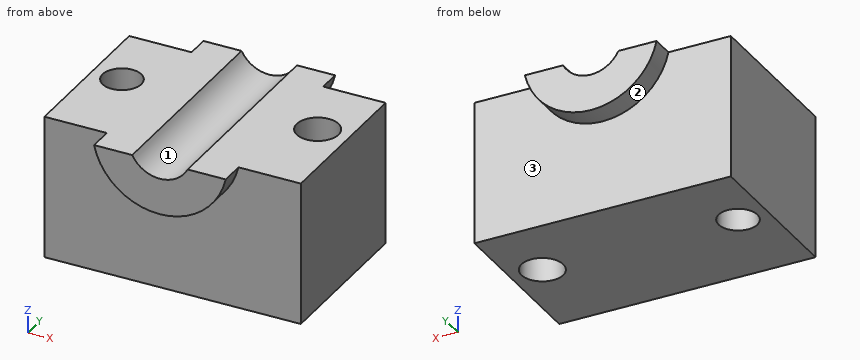
from build123d import *

# Parameters (mm, degrees)
F0_W          = 120.6022500992
F0_H          = 73.8097429276
F1_DEPTH      = 76.2
F2_R          = 31.6774975882
F3_DEPTH      = 86.868
F3_DEPTH_BACK = 11.43
F4_W          = 119.1478464752
F4_H          = 40.1731412858
F5_DEPTH      = 60.3021250496
F5_DEPTH_BACK = 60.3021250496
F6_R          = 14.6367961648
F7_DEPTH      = 86.869
F7_DEPTH_BACK = 25.4
F8_R          = 9.1115926715
F8_R_2        = 9.8364729175
F9_DEPTH      = 30.6065564433
F9_DEPTH_BACK = 36.9058714638


with BuildPart() as f1:
    # F0 (on Front) → F1 (new body)
    with BuildSketch(Plane.XZ):
        Rectangle(F0_W, F0_H)
    extrude(amount=-F1_DEPTH)

    # F2 (on Front) → F3 (join, two sides)
    with BuildSketch(Plane.XZ) as f3_sk:
        with Locations((0, 37.2918173671)):
            Circle(F2_R)
    extrude(amount=-F3_DEPTH)
    extrude(f3_sk.sketch, amount=F3_DEPTH_BACK)

    # F4 (on Right) → F5 (cut, two sides)
    with BuildSketch(Plane.YZ) as f5_sk:
        with Locations((41.5653018281, 50.6921270862)):
            Rectangle(F4_W, F4_H)
    extrude(amount=-F5_DEPTH, mode=Mode.SUBTRACT)
    extrude(f5_sk.sketch, amount=F5_DEPTH_BACK, mode=Mode.SUBTRACT)

    # F6 (on Front) → F7 (cut, two sides)
    with BuildSketch(Plane.XZ) as f7_sk:
        with Locations((0, 37.2918173671)):
            Circle(F6_R)
    extrude(amount=-F7_DEPTH, mode=Mode.SUBTRACT)
    extrude(f7_sk.sketch, amount=F7_DEPTH_BACK, mode=Mode.SUBTRACT)

    # F8 (on Top) → F9 (cut, two sides)
    with BuildSketch(Plane.XY) as f9_sk:
        with Locations((-46.2026000023, 42.7655205131)):
            Circle(F8_R)
        with Locations((45.4613789916, 43.5067377985)):
            Circle(F8_R_2)
    extrude(amount=F9_DEPTH, mode=Mode.SUBTRACT)
    extrude(f9_sk.sketch, amount=-F9_DEPTH_BACK, mode=Mode.SUBTRACT)


solid = f1.part
CAD build for the part. Positions are in the model's coordinates, mm. Face numbers are marked on the shaded views. Give positions to 0.01 mm unless a question says otherwise; leave off trailing zeros. Write each loop counter-clockwise with the first axis right and the second up, starting at its lowest first coordinate (ties: lowest second). Pieces come first, ordered by that corner, then holes. Notation, with made-up numbers: (82.5, -37) -> (107.5, -37) arc R24 cw to (107.5, -27) -> close; hole circle Ø1 at (42.25, -39.5). An arc over 180 degrees is marked (long way). Return JSON: item names as keys, results as strings.
Item 1: Band-saw the part on A-A (z = 26). List the corners of the cut face in (x, y), then the cut area to 3 significant figures.
Answer below:
{"outline": "(-60.3, 0) -> (-29.6, 0) -> (-29.6, -11.43) -> (-9.31, -11.43) -> (-9.31, 86.87) -> (-29.6, 86.87) -> (-29.6, 76.2) -> (-60.3, 76.2) -> close; (9.31, -11.43) -> (29.6, -11.43) -> (29.6, 0) -> (60.3, 0) -> (60.3, 76.2) -> (29.6, 76.2) -> (29.6, 86.87) -> (9.31, 86.87) -> close; hole circle Ø18.22 at (-46.2, 42.77); hole circle Ø19.67 at (45.46, 43.51)", "area": "8,100 mm2"}
Item 2: Band-saw the part on D-D (z = 15). List the corners of the cut face in (x, y), then the cut area to 3 significant figures.
Answer below:
{"outline": "(-60.3, 0) -> (-22.51, 0) -> (-22.51, -11.43) -> (22.51, -11.43) -> (22.51, 0) -> (60.3, 0) -> (60.3, 76.2) -> (22.51, 76.2) -> (22.51, 86.87) -> (-22.51, 86.87) -> (-22.51, 76.2) -> (-60.3, 76.2) -> close; hole circle Ø18.22 at (-46.2, 42.77); hole circle Ø19.67 at (45.46, 43.51)", "area": "9,620 mm2"}
Item 3: Band-saw the part on C-C (x = 0). List the corners of the cut face in (y, z), then the cut area to 3 significant figures.
Answer below:
{"outline": "(-11.43, 5.61) -> (0, 5.61) -> (0, -36.9) -> (76.2, -36.9) -> (76.2, 5.61) -> (86.87, 5.61) -> (86.87, 22.66) -> (-11.43, 22.66) -> close", "area": "4,920 mm2"}
Item 4: Drop flat-ended pins along their axis: pin 1 (11 mm diameter, centred on x = -46.2, y = 42.77, fed in from +Z); pin 2 (2 mm diameter, centred on x = 7, y = 22, fed in from +Z); pin 3 (6 mm diameter, centred on x = -3.5, z = -19, fed in from -Y); pin 4 (12 mm diameter, centred on x = 8, z = 6.5, fed in from +Y). Give the stop position or say it passes through.
Answer below:
{"pin 1": "passes through", "pin 2": "stops at z = 25.03", "pin 3": "stops at y = 0", "pin 4": "stops at y = 86.87"}
Item 5: Band-saw the part on B-B (y = 48.5). List the corners of the cut face in (x, z), then the cut area to 3 significant figures.
Answer below:
{"outline": "(-60.3, -36.9) -> (-53.28, -36.9) -> (-53.28, 30.61) -> (-60.3, 30.61) -> close; (-39.12, -36.9) -> (36.99, -36.9) -> (36.99, 30.61) -> (13.02, 30.61) arc R14.64 cw to (-13.02, 30.61) -> (-39.12, 30.61) -> close; (53.94, -36.9) -> (60.3, -36.9) -> (60.3, 30.61) -> (53.94, 30.61) -> close", "area": "5,890 mm2"}
Item 6: Two-plate mould, pull along X, no slides. Class the marked faces 1, 2 and 3: +X half, -X half, draft (parallel to the pull), parting line (faces both ways), or undercut.
Answer below:
{"face 1": "undercut", "face 2": "parting line", "face 3": "draft"}
Item 7: Drill centre lines: probe 1 along X at (y, z) = (48, -9); probe 2 along Y at (x, z) = (26, -6); probe 3 along Y at (x, z) = (-54.5, 2.5). Where is each one in solid material? Low to high.
Answer below:
{"probe 1": "x = -60.3 to -53.66, -38.74 to 36.71, 54.21 to 60.3", "probe 2": "y = 0 to 76.2", "probe 3": "y = 0 to 39, 46.53 to 76.2"}
